from build123d import *

# Parameters (mm, degrees)
SKETCH037_W     = 120
SKETCH037_H     = 45
PAD008_DEPTH    = 3
SKETCH038_W     = 113.5
SKETCH038_H     = 40
PAD009_DEPTH    = 6
SKETCH039_R     = 1.4
POCKET026_DEPTH = 116.751
POCKET027_DEPTH = 376.952357
CHAMFER008_SIZE = 2
SKETCH036_W     = 105
SKETCH036_H     = 37
POCKET028_DEPTH = 6
CHAMFER009_SIZE = 2
CHAMFER010_SIZE = 1
CHAMFER011_SIZE = 1
CHAMFER012_SIZE = 2


with BuildPart() as part:
    # Sketch037 → Pad008 (new body)
    with BuildSketch(Plane.XZ):
        Rectangle(SKETCH037_W, SKETCH037_H)
    extrude(amount=PAD008_DEPTH)

    # Sketch038 (on Face6 of Pad008) → Pad009 (join)
    with BuildSketch(Plane.XZ.offset(3)):
        Rectangle(SKETCH038_W, SKETCH038_H)
    extrude(amount=PAD009_DEPTH)

    # Sketch039 (on Face8 of Pad009) → Pocket026 (cut, through all)
    with BuildSketch(Plane(origin=(56.75, 0, 0), x_dir=(0, 0, 1), z_dir=(1, 0, 0))):
        with Locations((0, 6)):
            Circle(SKETCH039_R)
    extrude(amount=-POCKET026_DEPTH, mode=Mode.SUBTRACT)

    # Sketch040 (on Face3 of Pocket026) → Pocket027 (cut, through all)
    with BuildSketch(Plane(origin=(60, 0, 0), x_dir=(0, 0, 1), z_dir=(1, 0, 0))):
        Polygon((-22.5, 3), (-17.875456, -3.604533), (-35.516254, -3.604533), align=None)
    pocket027 = extrude(amount=-POCKET027_DEPTH, mode=Mode.SUBTRACT)

    # Mirrored: Pocket027 across Sketch040 V_Axis
    add(pocket027.mirror(Plane(origin=(60, 0, 0), x_dir=(1, 0, 0), z_dir=(0, 0, 1))), mode=Mode.SUBTRACT)

    # Chamfer008
    chamfer008_edges = [part.edges().sort_by_distance(p)[0] for p in [
        (60, 0, 0),
        (-60, 0, 0),
    ]]
    chamfer(chamfer008_edges, length=CHAMFER008_SIZE)

    # Sketch036 → Pocket028 (cut)
    with BuildSketch(Plane.XZ.offset(9)):
        Rectangle(SKETCH036_W, SKETCH036_H)
    extrude(amount=-POCKET028_DEPTH, mode=Mode.SUBTRACT)

    # Chamfer009
    chamfer009_edges = [part.edges().sort_by_distance(p)[0] for p in [
        (-56.75, -6, -20),
    ]]
    chamfer(chamfer009_edges, length=CHAMFER009_SIZE)

    # Chamfer010
    chamfer010_edges = [part.edges().sort_by_distance(p)[0] for p in [
        (56.75, -6, -20),
    ]]
    chamfer(chamfer010_edges, length=CHAMFER010_SIZE)

    # Chamfer011
    chamfer011_edges = [part.edges().sort_by_distance(p)[0] for p in [
        (56.75, -6, 20),
    ]]
    chamfer(chamfer011_edges, length=CHAMFER011_SIZE)

    # Chamfer012
    chamfer012_edges = [part.edges().sort_by_distance(p)[0] for p in [
        (-56.75, -6, 20),
    ]]
    chamfer(chamfer012_edges, length=CHAMFER012_SIZE)


with BuildPart() as part_1:
    # Body003 placement: moved
    add(part.part.moved(Location((7, 30, 110))))


solid = part_1.part
Could you check a few things on this model? Use its own coordinates, in mm. A direction names the side the tool comes from. Round coordinates to 2 decimals unless told otherwise and drop trailing zeros. Order: outer loops, then holes, each group sorted by start corner. A loop starts at its lowest first (then second) coordinate and runs counter-clockwise, first axis right, second up. Notation, with made-up numbers: M 78.5,-38 L 98.5,-38 A23 ccw 98.5,1 Z; hole C 16,7.25 d1. An arc over 180 degrees is marked long. One line per item, written item: value.
(1) If we mould it in two halves opening along X, with no side actions, what happens to faces 5 (the flat face through (7.84, 28.479, 131.464)), 6 (the flat face through (66, 29, 110)), 7 (the flat face through (6, 24, 128.5))? For each: released by +X, released by -X, zero draft, split by the parting line, or undercut.
Ans:
face 5: zero draft
face 6: released by +X
face 7: undercut
(2) Imagine slicing it at A-A (y = 24). Write out the boundary of the cut face in (x, z).
Ans:
outline: M -49.75,92 L -47.75,90 L 62.75,90 L 63.75,91 L 63.75,108.6 L 59.5,108.6 L 59.5,91.5 L -45.5,91.5 L -45.5,108.6 L -49.75,108.6 Z; M -49.75,111.4 L -45.5,111.4 L -45.5,128.5 L 59.5,128.5 L 59.5,111.4 L 63.75,111.4 L 63.75,129 L 62.75,130 L -47.75,130 L -49.75,128 Z
(3) Imagine slicing it at B-B (z = 110). Write out the boundary of the cut face in (x, y).
Ans:
outline: M -53,27 L -49.75,27 L -49.75,25.4 L -45.5,25.4 L -45.5,27 L 59.5,27 L 59.5,25.4 L 63.75,25.4 L 63.75,27 L 67,27 L 67,28 L 65,30 L -51,30 L -53,28 Z; M -49.75,21 L -45.5,21 L -45.5,22.6 L -49.75,22.6 Z; M 59.5,21 L 63.75,21 L 63.75,22.6 L 59.5,22.6 Z
(4) I need wall thicknesses on line 1 along X through (y, z) = (26, 124); line 2 along Z through (x, y) = (47.5, 25.25); line 3 along Z through (x, y) = (-46.4, 24). Which ranges of each line are inside material? Lowest first, please. Write a range as from..to.
Ans:
line 1: x = -49.75..-45.5, 59.5..63.75
line 2: z = 90..91.5, 128.5..130
line 3: z = 90..108.6, 111.4..130
(5) Imagine slicing it at C-C (x = 32.5). Write out the boundary of the cut face in (y, z).
Ans:
outline: M 21,90 L 27,90 L 27,87.5 L 30,89.6 L 30,130.4 L 27,132.5 L 27,130 L 21,130 L 21,128.5 L 27,128.5 L 27,91.5 L 21,91.5 Z
(6) I'm going to push flat-ended pins straight in: P1, Ø2, axis at y = 24, z = 110, coming from the +X side; P2, Ø3, axis at y = 24, z = 110, coming from the -X side; P3, Ø3, axis at x = 13.5, y = 23, coming from the -Z side; P4, Ø3, axis at x = -18.5, y = 24.5, coming from the +Z side. Where does each tip first touch, or does it pass through?
Ans:
P1: passes through
P2: stops at x = -49.75
P3: stops at z = 90
P4: stops at z = 130
(7) Which directions (+Z, -Z, +X, -X, +Y, -Y) give clear straight access to the entire face, cutting with the end or side of a thin tool? Please do faces 1 (the flat face through (-48.76, 24.04, 128.99)), 2 (the flat face through (-48.76, 24.04, 91.01)), 3 (the flat face through (7, 24, 90)), 4 (the flat face through (6, 24, 91.5)).
Ans:
face 1: +Z, -X, -Y
face 2: -Z, -X, -Y
face 3: -Z, +X, -X, -Y
face 4: -Y
